```python
from build123d import *

# Parameters (mm, degrees)
F0_R     = 3.65
F0_R_2   = 2.75
F0_R_3   = 1.95
F1_DEPTH = 3
F2_DEPTH = 5
F3_SIZE2 = 2.5
F3_SIZE  = 0.5
F4_DEPTH = 0.2


with BuildPart() as f1:
    # F0 (on Top) → F1 (new body)
    with BuildSketch(Plane.XY):
        with Locations((-17.504408526, 0)):
            Circle(F0_R)
        with Locations((-17.504408526, 0)):
            Circle(F0_R_2, mode=Mode.SUBTRACT)
        with Locations((-17.504408526, 0)):
            Circle(F0_R_2)
        with Locations((-17.504408526, 0)):
            Circle(F0_R_3, mode=Mode.SUBTRACT)
    extrude(amount=-F1_DEPTH)

    # F0 (on Top) → F2 (join)
    with BuildSketch(Plane.XY):
        with Locations((-17.504408526, 0)):
            Circle(F0_R)
        with Locations((-17.504408526, 0)):
            Circle(F0_R_2, mode=Mode.SUBTRACT)
    extrude(amount=F2_DEPTH)

    # F3
    f3_edges = [f1.edges().sort_by_distance(p)[0] for p in [
        (-21.154409, 0, -3),
    ]]
    f3_side = f1.faces().sort_by_distance((-21.051171, 0, -3))[0]
    chamfer(f3_edges, length=F3_SIZE, length2=F3_SIZE2, reference=f3_side)

    # F0 (on Top) → F4 (join)
    with BuildSketch(Plane.XY):
        with Locations((-17.504408526, 0)):
            Circle(F0_R_2)
        with Locations((-17.504408526, 0)):
            Circle(F0_R_3, mode=Mode.SUBTRACT)
        with Locations((-17.504408526, 0)):
            Circle(F0_R_3)
    extrude(amount=F4_DEPTH)


solid = f1.part
```
Can you work these out from the model? Positions are in its coordinate system, mm. A direction names the side the tool comes from. Round coordinates to 2 decimals unless told otherwise and drop trailing zeros. Loops run counter-clockwise (first coordinate to the right, second up) from the corner with the lowest first, then second, coordinate; pieces in that order, holes last. Notation, with made-up numbers: M 89.25,-3.5 L 95.25,-3.5 A19 ccw 95.25,0.5 Z; hole C 10,78.5 d10. An arc over 180 degrees is marked long. Answer in a Markdown table with one row per item.
1. If we section it at C-C, the plane z = -1.25: Please give me the cut outline in (x, y).
Established:
| item | result |
|---|---|
| outline | C -17.5,0 d7; hole C -17.5,0 d3.9 |
2. Please list where these lines run through material, in increasing order: line 1 (Z direction, x = -18, y = 0); line 2 (X direction, y = 0.25, z = 4.25); line 3 (Y direction, x = -18.75, z = 3.75). Write a range as from..to.
Established:
| item | result |
|---|---|
| line 1 | 0..0.2 |
| line 2 | -21.15..-20.24, -14.77..-13.86 |
| line 3 | -3.43..-2.45, 2.45..3.43 |
3. I'm going to push flat-ended pins straight in: pin 1 Ø3 at (x, y) = (-17.5, 0) entering from +Z; pin 2 Ø1.5 at (y, z) = (2.5, 0.5) entering from -X. Where does each tip first touch, or does it pass through?
Established:
| item | result |
|---|---|
| pin 1 | z = 0.2 |
| pin 2 | x = -20.71 |
4. If we section it at A-A, the plane y = 0: Please give me the cut outline in (x, z).
Established:
| item | result |
|---|---|
| outline | M -21.15,-0.5 L -20.65,-3 L -19.45,-3 L -19.45,0 L -15.55,0 L -15.55,-3 L -14.35,-3 L -13.85,-0.5 L -13.85,5 L -14.75,5 L -14.75,0.2 L -20.25,0.2 L -20.25,5 L -21.15,5 Z |
5. On a 3-axis mill with a long thin cutter (end or side, diameter ignored), from which of +Z, -Z, +X, -X, +Y, -Y can I reach the whole of each face in a straight line? I mean faces 5 (the face through (-20.25, 0.12, 2.57)), 6 (the face through (-15, 0, -3)). Say none if no direction works.
Established:
| item | result |
|---|---|
| face 5 | +Z |
| face 6 | -Z, +X, -X, +Y, -Y |
6. Thinking about a two-plate mould opening in X: for faces 1 (the face through (-18, 0, 0)), 2 (the face through (-14.023, 1.096, 2.288)), 3 (the face through (-15.644, 0.586, -1.479)), 4 (the face through (-17, 3, 5)), which applies, pulls with the +X half, pulls with the -X half, needs draft (parallel to the pull), parting line crosses it, or undercut?
Established:
| item | result |
|---|---|
| face 1 | undercut |
| face 2 | parting line crosses it |
| face 3 | undercut |
| face 4 | needs draft |
7. If we section it at B-B, the plane z = 2.5: Please give me the cut outline in (x, y), plus the area to 3 significant figures.
Established:
| item | result |
|---|---|
| outline | C -17.5,0 d7.3; hole C -17.5,0 d5.5 |
| area | 18.1 mm² |
